```python
from build123d import *

# Parameters (mm, degrees)
F0_W     = 20
F0_H     = 20
F1_DEPTH = 50
F2_W     = 10
F2_H     = 10
F3_DEPTH = 25
F4_W     = 10
F4_H     = 10
F5_DEPTH = 25
F6_W     = 10
F6_H     = 10
F7_DEPTH = 25


with BuildPart() as f1:
    # F0 (on Front) → F1 (new body)
    with BuildSketch(Plane.XZ):
        with Locations((-10, 10)):
            Rectangle(F0_W, F0_H)
    extrude(amount=F1_DEPTH)

    # F2 (on face) → F3 (cut)
    with BuildSketch(Plane.XZ.offset(50)):
        with Locations((-10, 10)):
            Rectangle(F2_W, F2_H)
    extrude(amount=-F3_DEPTH, mode=Mode.SUBTRACT)

    # F4 (on face) → F5 (cut)
    with BuildSketch(Plane.XY.offset(20)):
        with Locations((-10, -35)):
            Rectangle(F4_W, F4_H)
    extrude(amount=-F5_DEPTH, mode=Mode.SUBTRACT)

    # F6 (on face) → F7 (cut)
    with BuildSketch(Plane(origin=(-20, 0, 0), x_dir=(0, -1, 0), z_dir=(-1, 0, 0))):
        with Locations((35, 10)):
            Rectangle(F6_W, F6_H)
    extrude(amount=-F7_DEPTH, mode=Mode.SUBTRACT)


solid = f1.part
```
Verification items for the finished model (mm, model axes). A direction names the side the tool comes from. Coordinates: 2 decimals unless noted, no trailing zeros. Order: outer loops, then holes, each group sorted by start corner. A loop starts at its lowest first (then second) coordinate and runs counter-clockwise, first axis right, second up. Notation, with made-up numbers: (-30.5, 87.25) -> (3.5, 87.25) arc R21 cw to (3.5, 97.25) -> close; hole circle Ø2 at (51.5, -26). An arc over 180 degrees is marked (long way). Put each result on its own line as item: value. Start each with the question number.
1) Material ranges on L1, parallel to Y at x = -3, z = 9; L2, parallel to X at y = -42, z = 10.5; L3, parallel to Z at x = -6.5, y = -27.5, recorded low to high.
2) Cross-section at C-C (x = -10.75). Enter the section's corners in (y, z).
3) Tool access check on faces 1 (the flat face through (-3, -35, 5)), 2 (the flat face through (-20, -25, 10)), 3 (the flat face through (-10, -45, 15)), 4 (the flat face through (-5, -35, 3)), 5 (the flat face through (-10, -25, 0)). Record the directions out of +Z, -Z, +X, -X, +Y, -Y that give a thin tool (end or side, any length) a straight path to the whole face; none if there is none.
4) Cross-section at D-D (z = 8.25). Enter the section's corners in (x, y).
5) Cross-section at B-B (y = -29). Enter the section's corners in (x, z), plus the area to 3 significant figures.
6) Release check for a two-part mould opening along Y. For faces 6 (the flat face through (-10, -28, 5)), 7 (the flat face through (-3, -35, 15)), 8 (the flat face through (-10, 0, 10)) record: pulls with the +Y half, pulls with the -Y half, needs draft (parallel to the pull), parting line crosses it, or undercut.
7) Cross-section at A-A (z = 17). Enter the section's corners in (x, y).
8) Go/stop test with flat-tipped pins: pin 1 (3 mm diameter, centred on x = -8, z = 8.5, fed in from -Y); pin 2 (12 mm diameter, centred on x = -7, z = 17.5, fed in from +Y). Record where each tip stops, or that it passes through.
Geometry check:
1. L1: y = -50 to -40, -30 to 0
1. L2: x = -20 to -15, -5 to 0
1. L3: z = 0 to 5, 15 to 20
2. outline: (-50, 0) -> (-40, 0) -> (-40, 5) -> (-50, 5) -> close; (-50, 15) -> (-40, 15) -> (-40, 20) -> (-50, 20) -> close; (-30, 0) -> (0, 0) -> (0, 20) -> (-30, 20) -> (-30, 15) -> (-25, 15) -> (-25, 5) -> (-30, 5) -> close
3. face 1: +X, -X
3. face 2: +Z, -Z, -X, +Y, -Y
3. face 3: -Y
3. face 4: +Z, -Z
3. face 5: -Z, +X, -X, +Y, -Y
4. outline: (-20, -50) -> (-15, -50) -> (-15, -40) -> (-20, -40) -> close; (-20, -30) -> (-15, -30) -> (-15, -25) -> (-5, -25) -> (-5, -30) -> (0, -30) -> (0, 0) -> (-20, 0) -> close; (-5, -50) -> (0, -50) -> (0, -40) -> (-5, -40) -> close
5. outline: (-20, 0) -> (0, 0) -> (0, 20) -> (-20, 20) -> close; hole (-15, 5) -> (-5, 5) -> (-5, 15) -> (-15, 15) -> close
5. area: 300 mm^2
6. face 6: needs draft
6. face 7: undercut
6. face 8: pulls with the +Y half
7. outline: (-20, -50) -> (0, -50) -> (0, 0) -> (-20, 0) -> close; hole (-15, -40) -> (-5, -40) -> (-5, -30) -> (-15, -30) -> close
8. pin 1: stops at y = -25
8. pin 2: stops at y = 0
